```python
from build123d import *

# Parameters (mm, degrees)
SKETCH5_W          = 150
SKETCH5_H          = 150
CUT_EXTRUDE1_DEPTH = 100


with BuildPart() as part:
    # Sketch1 → Loft1 section 0
    with BuildSketch(Plane(origin=(0, 0, 0), x_dir=(1, 0, 0), z_dir=(0, 1, 0)), mode=Mode.PRIVATE) as loft1_s0:
        with BuildLine():
            Line((-500, -500), (500, -500))
            Line((500, -500), (500, 500))
            Line((500, 500), (-500, 500))
            Line((-500, 500), (-500, -500))
        make_face()
    loft([loft1_s0.sketch, Vertex(0, -400, 0)])

    # Sketch5 → Cut-Extrude1 (cut)
    with BuildSketch(Plane(origin=(0, -400, 0), x_dir=(-1, 0, 0), z_dir=(0, -1, 0))):
        Rectangle(SKETCH5_W, SKETCH5_H)
    extrude(amount=-CUT_EXTRUDE1_DEPTH, mode=Mode.SUBTRACT)


solid = part.part
```
For this review, take the finished solid that the model builds, in its own axes (mm). A direction names the side the tool comes from. Coordinates: 2 decimals unless noted, no trailing zeros. Order: outer loops, then holes, each group sorted by start corner. A loop starts at its lowest first (then second) coordinate and runs counter-clockwise, first axis right, second up. Notation, with made-up numbers: (33.25, 63.5) -> (69.25, 63.5) arc R24 cw to (69.25, 82.5) -> close; hole circle Ø10 at (1, -2). An arc over 180 degrees is marked (long way). Use CSV: the item, a comma, the result in double quotes. Start each with the question number.
Item 1: Wall thickness on probe 1 along Y at (x, z) = (-258, -180); probe 2 along X at (y, z) = (-289.5, -77.5) (3 decimals); probe 3 along Z at (x, y) = (-58.5, -242.5) (3 decimals): over which ranges is each line inside the solid? List them lowest first.
Item 2: Insertion check: pin 1 (12 mm diameter, centred on x = 11, y = -311, fed in from +Z); pin 2 (5 mm diameter, centred on x = -313, z = -248.5, fed in from -Y); pin 3 (12 mm diameter, centred on y = -230.5, z = -158.5, fed in from +X) (3 decimals); pin 4 (4 mm diameter, centred on x = 102.5, z = 143, fed in from +Y). Each pin has a flat end and moves straight along its axis. Give the tip position at first contact, or say it passes through.
Item 3: For faces 1 (the face through (1, -320, -75)), 2 (the face through (331.75, -134.6, 7)), list the 3-axis set-ups (+Z, -Z, +X, -X, +Y, -Y) from which the entire face can be reached by the end or side of a thin tool; tool diameter is ignored.
Item 4: We need section A-A, the plane y = -314. Give the boundary of the cut face in (x, z).
Item 5: Draft analysis for pull direction Z (two halves, no side actions). For faces 3 (the face through (0, 0, 14)), 4 (the face through (7, -134.6, -331.75)), 5 (the face through (-75, -320, 1)), state which applies: pulls with the +Z half, pulls with the -Z half, needs draft (parallel to the pull), parting line crosses it, or undercut.
Item 6: We need section C-C, the plane x = -324. Give the boundary of the cut face in (y, z), then the cut area to 3 significant figures.
Item 7: We need section D-D, the plane y = -187. Give the boundary of the cut face in (x, z).
Item 8: We need section B-B, the plane z = -55. Give the boundary of the cut face in (x, y), then the cut area to 4 significant figures.
Derived:
1,probe 1,"y = -193.6 to 0"
1,probe 2,"x = -138.125 to 138.125"
1,probe 3,"z = -196.875 to 196.875"
2,pin 1,"stops at z = 118.75"
2,pin 2,"stops at y = -151.6"
2,pin 3,"stops at x = 219.375"
2,pin 4,"stops at y = 0"
3,face 1,"-Y"
3,face 2,"+Z, -Z, +X, -Y"
4,outline,"(-107.5, -107.5) -> (107.5, -107.5) -> (107.5, 107.5) -> (-107.5, 107.5) -> close; hole (-75, -75) -> (75, -75) -> (75, 75) -> (-75, 75) -> close"
5,face 3,"needs draft"
5,face 4,"pulls with the -Z half"
5,face 5,"undercut"
6,outline,"(-140.8, -324) -> (0, -500) -> (0, 500) -> (-140.8, 324) -> close"
6,area,"116,000 mm^2"
7,outline,"(-266.25, -266.25) -> (266.25, -266.25) -> (266.25, 266.25) -> (-266.25, 266.25) -> close"
8,outline,"(-500, 0) -> (-75, -340) -> (-75, -300) -> (75, -300) -> (75, -340) -> (500, 0) -> close"
8,area,"189,500 mm^2"
